from build123d import *

# Parameters (mm, degrees)
SKETCH3_R           = 5
BOSS_EXTRUDE1_DEPTH = 6.25
FILLET1_R           = 1
SKETCH5_R           = 4
BOSS_EXTRUDE3_DEPTH = 8.75
SKETCH4_R           = 4
BOSS_EXTRUDE4_DEPTH = 8.75
SKETCH6_R           = 2.5
CUT_EXTRUDE3_DEPTH  = 6
SKETCH7_R           = 2.5
CUT_EXTRUDE4_DEPTH  = 6
BOSS_EXTRUDE5_START = -2.5
SKETCH8_R           = 5
SKETCH8_R_2         = 2.5
BOSS_EXTRUDE5_DEPTH = 2.5
SKETCH9_R           = 5
SKETCH9_R_2         = 2.5
BOSS_EXTRUDE6_DEPTH = 2.5
CHAMFER1_SIZE       = 0.5


with BuildPart() as part:
    # Sketch3 → Boss-Extrude1 (new, symmetric)
    with BuildSketch(Plane(origin=(0, 0, 0), x_dir=(1, 0, 0), z_dir=(0, 1, 0))):
        with Locations(Location((0, 0, 0), (0, 0, 270))):
            Circle(SKETCH3_R)
    extrude(amount=BOSS_EXTRUDE1_DEPTH, both=True)

    # Fillet1
    fillet1_edges = [part.edges().sort_by_distance(p)[0] for p in [
        (0, -6.25, -5),
        (0, 6.25, -5),
    ]]
    fillet(fillet1_edges, radius=FILLET1_R)

    # Sketch5 → Boss-Extrude3 (add, symmetric)
    with BuildSketch(Plane.XY):
        with Locations(Location((0, 0, 0), (0, 0, 180))):
            Circle(SKETCH5_R)
    extrude(amount=BOSS_EXTRUDE3_DEPTH, both=True)

    # Sketch4 → Boss-Extrude4 (add, symmetric)
    with BuildSketch(Plane(origin=(0, 0, 0), x_dir=(0, 0, -1), z_dir=(1, 0, 0))):
        with Locations(Location((0, 0, 0), (0, 0, 207.885566817))):
            Circle(SKETCH4_R)
    extrude(amount=BOSS_EXTRUDE4_DEPTH, both=True)

    # Sketch6 → Cut-Extrude3 (cut)
    with BuildSketch(Plane(origin=(8.75, 0, 0), x_dir=(0, 0, -1), z_dir=(1, 0, 0))):
        Circle(SKETCH6_R)
    cut_extrude3 = extrude(amount=-CUT_EXTRUDE3_DEPTH, mode=Mode.SUBTRACT)

    # Sketch7 → Cut-Extrude4 (cut)
    with BuildSketch(Plane(origin=(0, 0, -8.75), x_dir=(-1, 0, 0), z_dir=(0, 0, -1))):
        Circle(SKETCH7_R)
    cut_extrude4 = extrude(amount=-CUT_EXTRUDE4_DEPTH, mode=Mode.SUBTRACT)

    # Sketch8 → Boss-Extrude5 (add)
    with BuildSketch(Plane.ZY.offset(8.75).offset(BOSS_EXTRUDE5_START)):
        Circle(SKETCH8_R)
        with Locations(Location((0, 0, 0), (0, 0, 180))):
            Circle(SKETCH8_R_2, mode=Mode.SUBTRACT)
    boss_extrude5 = extrude(amount=BOSS_EXTRUDE5_DEPTH)

    # Mirror1: Boss-Extrude5 across plane
    add(boss_extrude5.mirror(Plane(origin=(0, 0, 0), x_dir=(0, 0, 1), z_dir=(1, 0, 0))))

    # Sketch9 → Boss-Extrude6 (add)
    with BuildSketch(Plane(origin=(0, 0, -8.75), x_dir=(-1, 0, 0), z_dir=(0, 0, -1))):
        Circle(SKETCH9_R)
        Circle(SKETCH9_R_2, mode=Mode.SUBTRACT)
    boss_extrude6 = extrude(amount=-BOSS_EXTRUDE6_DEPTH)

    # Mirror2: Boss-Extrude6 across plane
    add(boss_extrude6.mirror(Plane.XY))

    # Mirror3: Cut-Extrude3 across plane
    add(cut_extrude3.mirror(Plane(origin=(0, 0, 0), x_dir=(0, 0, 1), z_dir=(1, 0, 0))), mode=Mode.SUBTRACT)

    # Mirror4: Cut-Extrude4 across plane
    add(cut_extrude4.mirror(Plane.XY), mode=Mode.SUBTRACT)

    # Chamfer1
    chamfer1_edges = [part.edges().sort_by_distance(p)[0] for p in [
        (-6.25, 0, -5),
        (-8.75, 0, -5),
        (6.25, 0, -5),
        (8.75, 0, -5),
        (5, 0, -8.75),
        (5, 0, -6.25),
        (5, 0, 6.25),
        (5, 0, 8.75),
    ]]
    chamfer(chamfer1_edges, length=CHAMFER1_SIZE)


solid = part.part
Read the model definition and answer for the solid it produces. Units are mm, in the model's axes. A direction names the side the tool comes from. Round coordinates to 2 decimals unless told otherwise and drop trailing zeros. Loops run counter-clockwise (first coordinate to the right, second up) from the corner with the lowest first, then second, coordinate; pieces in that order, holes last. Notation, with made-up numbers: (9, 0.25) - (26, 0.25) arc R19 ccw to (26, 6.25) - close; hole circle Ø3 at (67.5, -29.75). An arc over 180 degrees is marked (long way). One line per question, with ' | ' between items. Start each with the question number.
Q1. Flat-ended cylindrical pins translate along their axes: pin 1 (6 mm diameter, centred on x = 2, y = 4.5, fed in from +Z); pin 2 (3 mm diameter, centred on y = 0, z = 0, fed in from +X); pin 3 (1.5 mm diameter, centred on y = 0.5, z = -0.5, fed in from -X); pin 4 (2 mm diameter, centred on x = -6.5, z = 2.5, fed in from +Y). Find the tip coordinate at first contact, or state that the pin passes through.
Q2. For faces 4 (the flat face through (0, 0, -2.75)), 5 (the flat face through (6.25, -3, -3)), 6 (the cylindrical face through (-5.79, -2.44, 0.54)), 7 (the flat face through (2.75, 0, 0)), determine the directions among +Z, -Z, +X, -X, +Y, -Y from which every point of the face is accessible in a straight line to the end or side of a thin tool.
Q3. For a pull along Y with two mould halves and no side action, classify faces 1 (the flat face through (-8.75, -2, 2)), 2 (the flat face through (0, 6.25, 0)), 3 (the cylindrical face through (0.54, -2.44, -5.79)) as +Y half, -Y half, draft (parallel to the pull), parting line (faces both ways), or undercut.
Q4. Section A-A on z = 4.75 is taken. Count the separate pieces of the cut face and the enclosed holes in it, plus the area to 3 significant figures.
Q5. Find the intervals of material crossed by L1, parallel to Y at x = 7.35, z = 0; L2, parallel to Y at x = -5.9, z = 0; L3, parallel to X at y = 4, z = -0.5, in increasing order.
Q6. Section B-B on x = 7.25 is taken. Give the vertices of the cut face in (y, z), plus the area to 3 significant figures.
Established:
1) pin 1: z = 8.75 | pin 2: x = 2.75 | pin 3: x = -2.75 | pin 4: y = 4.76
2) face 4: -Z | face 5: none | face 6: -X | face 7: +X
3) face 1: draft | face 2: +Y half | face 3: undercut
4) separate pieces: 3 | enclosed holes: 1 | area: 53.8 mm²
5) L1: -5 to -2.5, 2.5 to 5 | L2: -4 to -2.5, 2.5 to 4 | L3: -8.75 to -6.25, -4.97 to 4.97, 6.25 to 8.75
6) outline: circle Ø10 at (0, 0); hole circle Ø5 at (0, 0) | area: 58.9 mm²
